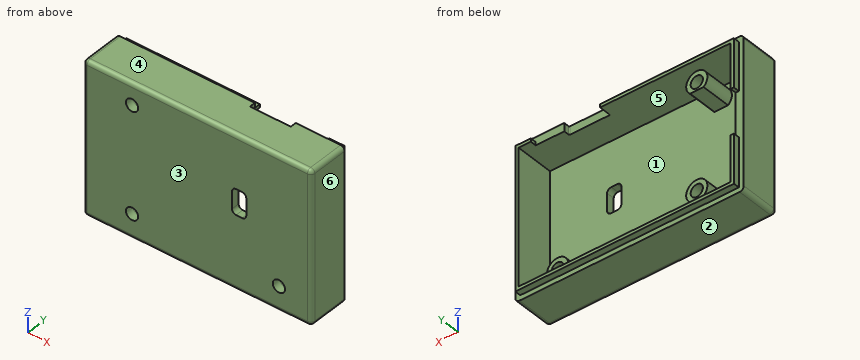
```python
from build123d import *

# Parameters (mm, degrees)
SKETCH1_W           = 56
SKETCH1_H           = 37.25
BOSS_EXTRUDE1_DEPTH = 2
SKETCH2_W           = 56
SKETCH2_H           = 37.25
SKETCH2_W_2         = 52
SKETCH2_H_2         = 33.25
BOSS_EXTRUDE2_DEPTH = 9
SKETCH3_R           = 2.6
SKETCH3_R_2         = 1.5
BOSS_EXTRUDE3_DEPTH = 7.4
SKETCH5_W           = 56
SKETCH5_H           = 37.25
SKETCH5_W_2         = 53.6
SKETCH5_H_2         = 34.85
CUT_EXTRUDE1_DEPTH  = 1
FILLET1_R           = 1
SKETCH7_R           = 1.5
CUT_EXTRUDE2_DEPTH  = 10
CUT_EXTRUDE3_DEPTH  = 3
FILLET2_R           = 1
CUT_EXTRUDE4_DEPTH  = 7.4
SKETCH10_W          = 3.5
SKETCH10_H          = 6.2
CUT_EXTRUDE5_DEPTH  = 10
FILLET3_R           = 1
SKETCH11_W          = 7
SKETCH11_H          = 1
CUT_EXTRUDE6_DEPTH  = 10
FILLET4_R           = 0.2
BOSS_EXTRUDE6_DEPTH = 0.5
SKETCH13_W          = 11.063396545
SKETCH13_H          = 1.5
CUT_EXTRUDE9_DEPTH  = 2
SKETCH14_R          = 2.6
CUT_EXTRUDE10_DEPTH = 2.3


with BuildPart() as part:
    # Sketch1 → Boss-Extrude1 (new body)
    with BuildSketch(Plane(origin=(0, 0, 0), x_dir=(1, 0, 0), z_dir=(0, 1, 0))):
        with Locations((28, 18.625)):
            Rectangle(SKETCH1_W, SKETCH1_H)
    extrude(amount=BOSS_EXTRUDE1_DEPTH)

    # Sketch2 → Boss-Extrude2 (add)
    with BuildSketch(Plane(origin=(0, 2, 0), x_dir=(1, 0, 0), z_dir=(0, 1, 0))):
        with Locations((28, 18.625)):
            Rectangle(SKETCH2_W, SKETCH2_H)
        with Locations((28, 18.625)):
            Rectangle(SKETCH2_W_2, SKETCH2_H_2, mode=Mode.SUBTRACT)
    extrude(amount=BOSS_EXTRUDE2_DEPTH)

    # Sketch3 → Boss-Extrude3 (add)
    with BuildSketch(Plane(origin=(0, 2, 0), x_dir=(1, 0, 0), z_dir=(0, 1, 0))):
        with Locations((12, 5.25)):
            Circle(SKETCH3_R)
        with Locations((12, 5.25)):
            Circle(SKETCH3_R_2, mode=Mode.SUBTRACT)
        with Locations((12, 31.25)):
            Circle(SKETCH3_R)
        with Locations((12, 31.25)):
            Circle(SKETCH3_R_2, mode=Mode.SUBTRACT)
        with Locations((48, 31.25)):
            Circle(SKETCH3_R)
        with Locations((48, 31.25)):
            Circle(SKETCH3_R_2, mode=Mode.SUBTRACT)
    extrude(amount=BOSS_EXTRUDE3_DEPTH)

    # Sketch5 → Cut-Extrude1 (cut)
    with BuildSketch(Plane(origin=(0, 11, 0), x_dir=(1, 0, 0), z_dir=(0, 1, 0))):
        with Locations((28, 18.625)):
            Rectangle(SKETCH5_W, SKETCH5_H)
        with Locations((28, 18.625)):
            Rectangle(SKETCH5_W_2, SKETCH5_H_2, mode=Mode.SUBTRACT)
    extrude(amount=-CUT_EXTRUDE1_DEPTH, mode=Mode.SUBTRACT)

    # Fillet1
    fillet1_edges = [part.edges().sort_by_distance(p)[0] for p in [
        (0, 5, -37.25),
        (56, 5, -37.25),
        (56, 5, 0),
        (0, 5, 0),
    ]]
    fillet(fillet1_edges, radius=FILLET1_R)

    # Sketch7 → Cut-Extrude2 (cut)
    with BuildSketch(Plane(origin=(0, 2, 0), x_dir=(1, 0, 0), z_dir=(0, 1, 0))):
        with Locations((12, 5.25)):
            Circle(SKETCH7_R)
        with Locations((48, 31.25)):
            Circle(SKETCH7_R)
        with Locations((12, 31.25)):
            Circle(SKETCH7_R)
    extrude(amount=-CUT_EXTRUDE2_DEPTH, mode=Mode.SUBTRACT)

    # Sketch8 → Cut-Extrude3 (cut)
    with BuildSketch(Plane.XY):
        Polygon((44, 10), (44, 8.5), (34, 8.5), (34, 10), (34, 11), (44, 11), align=None)
    extrude(amount=-CUT_EXTRUDE3_DEPTH, mode=Mode.SUBTRACT)

    # Fillet2
    fillet2_edges = [part.edges().sort_by_distance(p)[0] for p in [
        (28, 0, -37.25),
        (0, 0, -18.625),
        (56, 0, -18.625),
        (28, 0, 0),
        (0.292893219, 0, -0.292893219),
        (0.292893219, 0, -36.957106781),
        (55.707106781, 0, -0.292893219),
        (55.707106781, 0, -36.957106781),
    ]]
    fillet(fillet2_edges, radius=FILLET2_R)

    # Sketch9 → Cut-Extrude4 (cut)
    with BuildSketch(Plane(origin=(0, 9.4, 0), x_dir=(1, 0, 0), z_dir=(0, 1, 0))):
        with BuildLine():
            Line((12, 7.25), (13.661324773, 7.25))
            ThreePointArc((13.661324773, 7.25), (12, 7.85), (10.338675227, 7.25))
            Line((10.338675227, 7.25), (12, 7.25))
        make_face()
    extrude(amount=-CUT_EXTRUDE4_DEPTH, mode=Mode.SUBTRACT)

    # Sketch10 → Cut-Extrude5 (cut)
    with BuildSketch(Plane(origin=(0, 2, 0), x_dir=(1, 0, 0), z_dir=(0, 1, 0))):
        with Locations((38.25, 16.15)):
            Rectangle(SKETCH10_W, SKETCH10_H)
    extrude(amount=-CUT_EXTRUDE5_DEPTH, mode=Mode.SUBTRACT)

    # Fillet3
    fillet3_edges = [part.edges().sort_by_distance(p)[0] for p in [
        (36.5, 1, -13.05),
        (36.5, 1, -19.25),
        (40, 1, -19.25),
        (40, 1, -13.05),
    ]]
    fillet(fillet3_edges, radius=FILLET3_R)

    # Sketch11 → Cut-Extrude6 (cut)
    with BuildSketch(Plane.XY.offset(-1.2)):
        with Locations((47.5, 10.5)):
            Rectangle(SKETCH11_W, SKETCH11_H)
    extrude(amount=-CUT_EXTRUDE6_DEPTH, mode=Mode.SUBTRACT)

    # Fillet4
    fillet4_edges = [part.edges().sort_by_distance(p)[0] for p in [
        (44, 8.5, -1),
        (34, 8.5, -1),
    ]]
    fillet(fillet4_edges, radius=FILLET4_R)

    # Sketch12 → Boss-Extrude6 (add)
    with BuildSketch(Plane(origin=(0, 11, 0), x_dir=(1, 0, 0), z_dir=(0, 1, 0))):
        Polygon((51, 2), (51, 1.2), (54.8, 1.2), (54.8, 36.05), (1.2, 36.05), (1.2, 1.2), (34, 1.2), (34, 2), (2, 2), (2, 35.25), (54, 35.25), (54, 2), align=None)
    extrude(amount=BOSS_EXTRUDE6_DEPTH)

    # Sketch13 → Cut-Extrude9 (cut)
    with BuildSketch(Plane.ZY.offset(-1.2)):
        with Locations((-18.511698272, 10.75)):
            Rectangle(SKETCH13_W, SKETCH13_H)
    extrude(amount=-CUT_EXTRUDE9_DEPTH, mode=Mode.SUBTRACT)

    # Sketch14 → Cut-Extrude10 (cut)
    with BuildSketch(Plane(origin=(0, 9.4, 0), x_dir=(1, 0, 0), z_dir=(0, 1, 0))):
        with Locations((48, 31.25)):
            Circle(SKETCH14_R)
    extrude(amount=-CUT_EXTRUDE10_DEPTH, mode=Mode.SUBTRACT)


solid = part.part
```
Design review of the part built by this model. Coordinates are the model's own, in mm. Face numbers are marked on the shaded views. A direction names the side the tool comes from. Coordinates: 2 decimals unless noted, no trailing zeros. Order: outer loops, then holes, each group sorted by start corner. A loop starts at its lowest first (then second) coordinate and runs counter-clockwise, first axis right, second up. Notation, with made-up numbers: (-36, -25.5) -> (1, -25.5) arc R37 ccw to (1, 11.5) -> close; hole circle Ø9 at (80.25, 86.5). An arc over 180 degrees is marked (long way). One line per item, written item: value. Start each with the question number.
Q1. Mouldability with a two-part tool opening along Z and no side actions: class the marked faces 1, 2, 3 and 4 as pulls with the +Z half, pulls with the -Z half, needs draft (parallel to the pull), parting line crosses it, or undercut.
Q2. Insertion check: pin 1 Ø2.5 at (x, z) = (12, -5.25) entering from +Y; pin 2 Ø12 at (x, z) = (46, -10) entering from +Y; pin 3 Ø5 at (x, z) = (12, -5) entering from +Y; pin 4 Ø1 at (x, z) = (38, -1.5) entering from +Y. Each pin has a flat end and moves straight along its axis. Give the tip position at first contact, or say it passes through.
Q3. For probe 1 along X at (y, z) = (1.5, -31.25); probe 2 along X at (y, z) = (4.8, -31.25); probe 3 along Z at (x, y) = (12, 1), list the stretches that pass through material, from the lowest coordinate up.
Q4. Tool access review of the marked faces 5 and 6: name each direction out of +Z, -Z, +X, -X, +Y, -Y from which nothing blocks a thin tool from reaching the whole face with its end or side.
Q5. Take a section at C-C, the plane x = 48. State the section outline as (y, z) points.
Q6. Take a section at D-D, the plane z = -31.25. Give the number of separate pieces and of enclosed holes in the cut face, then the cut area to 3 significant figures.
Q7. Take a section at A-A, the plane y = 3.5. State the section outline as (x, z) points.
Q8. Take a section at B-B, the plane z = -5.25. State the section outline as (x, y) points, then the cut area to 3 significant figures.
Values follow:
1. face 1: undercut
1. face 2: pulls with the -Z half
1. face 3: needs draft
1. face 4: pulls with the +Z half
2. pin 1: passes through
2. pin 2: stops at y = 2
2. pin 3: stops at y = 9.4
2. pin 4: stops at y = 8.5
3. probe 1: x = 0 to 10.5, 13.5 to 46.5, 49.5 to 56
3. probe 2: x = 0 to 2, 9.4 to 10.5, 13.5 to 14.6, 45.4 to 46.5, 49.5 to 50.6, 54 to 56
3. probe 3: z = -37.25 to -32.75, -29.75 to -6.75, -3.75 to 0
4. face 5: +Y
4. face 6: +Z, -Z, +X, +Y, -Y
5. outline: (0, -36.25) arc R1 ccw to (1, -37.25) -> (10, -37.25) -> (10, -36.05) -> (11.5, -36.05) -> (11.5, -35.25) -> (2, -35.25) -> (2, -33.85) -> (7.1, -33.85) -> (7.1, -32.75) -> (0, -32.75) -> close; (0, -29.75) -> (7.1, -29.75) -> (7.1, -28.65) -> (2, -28.65) -> (2, -2) -> (10, -2) -> (10, 0) -> (1, 0) arc R1 ccw to (0, -1) -> close
6. separate pieces: 3
6. enclosed holes: 0
6. area: 161 mm2
7. outline: (0, -36.25) arc R1 ccw to (1, -37.25) -> (55, -37.25) arc R1 ccw to (56, -36.25) -> (56, -1) arc R1 ccw to (55, 0) -> (1, 0) arc R1 ccw to (0, -1) -> close; circle Ø5.2 at (12, -31.25); (10.34, -7.25) -> (13.66, -7.25) arc R2.6 ccw (long way) to start; circle Ø5.2 at (48, -31.25); hole (2, -35.25) -> (54, -35.25) -> (54, -2) -> (2, -2) -> close; hole circle Ø3 at (12, -31.25); hole circle Ø3 at (12, -5.25); hole circle Ø3 at (48, -31.25)
8. outline: (0, 1) arc R1 ccw to (1, 0) -> (10.5, 0) -> (10.5, 9.4) -> (9.4, 9.4) -> (9.4, 2) -> (2, 2) -> (2, 11.5) -> (1.2, 11.5) -> (1.2, 10) -> (0, 10) -> close; (13.5, 0) -> (55, 0) arc R1 ccw to (56, 1) -> (56, 10) -> (54.8, 10) -> (54.8, 11.5) -> (54, 11.5) -> (54, 2) -> (14.6, 2) -> (14.6, 9.4) -> (13.5, 9.4) -> close
8. area: 156 mm2
